Part model, mm, in its own coordinate system. Face numbers are marked on the shaded views. A direction names the side the tool comes from. Round coordinates to 2 decimals unless told otherwise and drop trailing zeros. Write each loop counter-clockwise with the first axis right and the second up, starting at its lowest first coordinate (ties: lowest second). Pieces come first, ordered by that corner, then holes. Notation, with made-up numbers: M 22,12 L 28,12 A33 cw 28,46 Z; hole C 59,-6 d1. An arc over 180 degrees is marked long. One line per question, with ' | ' between items. Start each with the question number.
1) Saw through at C-C (x = -16). List the corners of the cut face in (y, z), plus the area to 3 significant figures.
2) Saw through at A-A (y = 0). List the corners of the cut face in (x, z), plus the area to 3 significant figures.
3) Saw through at D-D (x = 2.5). List the corners of the cut face in (y, z), plus the area to 3 significant figures.
4) Mould opens along Y. For the marked faces 1, 2 and 3 say: pulls with the +Y half, pulls with the -Y half, needs draft (parallel to the pull), parting line crosses it, or undercut.
5) Wall check: probe 1 along Z at (x, y) = (9.5, -16); probe 2 along X at (y, z) = (4.5, 6.5); probe 3 along Y at (x, z) = (1.5, 8). Give the ranges that are in metal, low to high. Write a range as [from, to].
6) Drop flat-ended pins along their axis: pin 1 Ø8 at (x, z) = (-8, 43.5) entering from -Y; pin 2 Ø1 at (y, z) = (12.5, 15) entering from -X; pin 3 Ø8 at (y, z) = (-20, 26) entering from +X. Give the stop position or say it passes through.
7) Tool access for the marked faces 4, 5 and 6: list every direction of +Z, -Z, +X, -X, +Y, -Y with a clear straight run to the whole face (end or side of a thin tool).
8) Saw through at B-B (z = 46.5). List the corners of the cut face in (x, y), plus the area to 3 significant figures.
Autodesk Inventor part; units mm, degrees
ref_plane "YZ Plane" through (0, 0, 0) normal (1, 0, 0) x (0, 1, 0)
ref_plane "XZ Plane" through (0, 0, 0) normal (0, 1, 0) x (-1, 0, 0)
ref_plane "XY Plane" through (0, 0, 0) normal (0, 0, 1) x (1, 0, 0)
sketch "Sketch1" plane through (0, 0, 0) normal (0, 0, 1) x (1, 0, 0)
  circle A0 centre (0, 0) radius 17.526
  dimension "d0" = 35.052
extrude "Extrusion1" add sketch "Sketch1" along normal blind 38.1
sketch "Sketch2" plane through (0, 0, 38.1) normal (0, 0, 1) x (1, 0, 0)
  circle A0 centre (0, 0) radius 25.4
  dimension "d3" = 50.8
extrude "Extrusion2" add sketch "Sketch2" along normal blind 12.7
sketch "Sketch3" plane through (0, 0, 50.8) normal (0, 0, 1) x (1, 0, 0)
  line L0 (0, -7.3406) -> (-6.3571, -3.6703)
  line L1 (-6.3571, -3.6703) -> (-6.3571, 3.6703)
  line L2 (-6.3571, 3.6703) -> (0, 7.3406)
  line L3 (0, 7.3406) -> (6.3571, 3.6703)
  line L4 (6.3571, 3.6703) -> (6.3571, -3.6703)
  line L5 (6.3571, -3.6703) -> (0, -7.3406)
  point P0 (0, 0)
  point P1 (0, 0)
  dimension "d7" = 14.6812
extrude "Extrusion3" cut sketch "Sketch3" against normal through all
properties part number "Hex Adapter" material "PC/ABS Plastic"
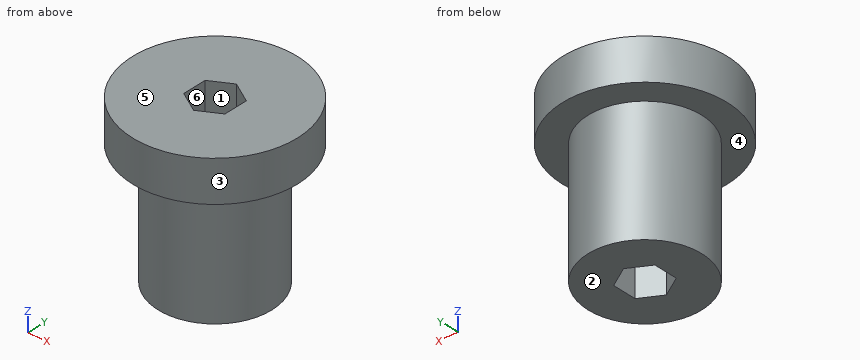
Answer key:
1) outline: M -19.73,38.1 L -7.15,38.1 L -7.15,0 L 7.15,0 L 7.15,38.1 L 19.73,38.1 L 19.73,50.8 L -19.73,50.8 Z | area: 1,050 mm2
2) outline: M -25.4,38.1 L -17.53,38.1 L -17.53,0 L -6.36,0 L -6.36,50.8 L -25.4,50.8 Z; M 6.36,0 L 17.53,0 L 17.53,38.1 L 25.4,38.1 L 25.4,50.8 L 6.36,50.8 Z | area: 1,330 mm2
3) outline: M -25.28,38.1 L -17.35,38.1 L -17.35,0 L -5.9,0 L -5.9,50.8 L -25.28,50.8 Z; M 5.9,0 L 17.35,0 L 17.35,38.1 L 25.28,38.1 L 25.28,50.8 L 5.9,50.8 Z | area: 1,360 mm2
4) face 1: undercut | face 2: needs draft | face 3: parting line crosses it
5) probe 1: z = [38.1, 50.8] | probe 2: x = [-16.94, -4.92], [4.92, 16.94] | probe 3: y = [-17.46, -6.47], [6.47, 17.46]
6) pin 1: stops at y = -25.08 | pin 2: stops at x = -12.77 | pin 3: stops at x = 7.15
7) face 4: -Z | face 5: +Z, +X, -X, +Y, -Y | face 6: +Z, -Z
8) outline: C 0,0 d50.8; hole M -6.36,-3.67 L 0,-7.34 L 6.36,-3.67 L 6.36,3.67 L 0,7.34 L -6.36,3.67 Z | area: 1,890 mm2
